Model file for the job. Use its own axes, mm. A direction names the side the tool comes from. Give positions to 0.01 mm unless a question says otherwise; leave off trailing zeros. Loops run counter-clockwise (first coordinate to the right, second up) from the corner with the lowest first, then second, coordinate; pieces in that order, holes last. Notation, with made-up numbers: (78, 11.5) - (85, 11.5) arc R26 ccw to (85, 31.5) - close; hole circle Ø11 at (11, 2). An arc over 180 degrees is marked (long way). Use a Markdown table: item, result.
from build123d import *

# Parameters (mm, degrees)
BOSS_EXTRUDE1_DEPTH         = 4.159999906
TAP_DRILL_FOR_M5X0_8_TAP1_D = 4.2
SKETCH8_W                   = 0.52
SKETCH8_H                   = 0.81


with BuildPart() as part:
    # Sketch1 → Boss-Extrude1 (new body)
    with BuildSketch(Plane(origin=(0, 0, 0), x_dir=(1, 0, 0), z_dir=(0, 1, 0))):
        Polygon((-4, -2.309401077), (0, -4.618802154), (4, -2.309401077), (4, 2.309401077), (0, 4.618802154), (-4, 2.309401077), align=None)
    extrude(amount=BOSS_EXTRUDE1_DEPTH)

    # Sketch3 → Revolve1 (revolve)
    with BuildSketch(Plane.XY):
        with BuildLine():
            Line((3.17, 4.989999906), (0, 4.989999906))
            Line((0, 4.989999906), (0, 4.159999906))
            Line((0, 4.159999906), (4, 4.159999906))
            ThreePointArc((4, 4.159999906), (3.756898628, 4.746898534), (3.17, 4.989999906))
        make_face()
    revolve(axis=Axis((0, 4.989999906, 0), (0, -1, 0)))

    # Tap Drill for M5x0.8 Tap1 (through all)
    with Locations(Plane(origin=(0, 0, 0), x_dir=(-1, 0, 0), z_dir=(0, -1, 0))):
        with Locations((0, 0)):
            Hole(TAP_DRILL_FOR_M5X0_8_TAP1_D / 2)

    # Sketch8 → Revolve2 (revolve)
    with BuildSketch(Plane.XY):
        with Locations((1.84, 4.554999966)):
            Rectangle(SKETCH8_W, SKETCH8_H)
    revolve(axis=Axis((0, 4.989999906, 0), (0, -1, 0)))


solid = part.part
(1) Pin check, flat tips, straight feed: P1, Ø0.6, axis at x = -3, z = -2, coming from the +Y side; P2, Ø2, axis at x = -2, y = 1, coming from the +Z side; P3, Ø1.3, axis at x = -0.5, z = 0.5, coming from the -Y side; P4, Ø0.9, axis at x = 0.5, z = 4, coming from the +Y side. Stop position of each tip, or through.
Computed:
| item | result |
|---|---|
| P1 | y = 4.98 |
| P2 | z = 4.04 |
| P3 | through |
| P4 | y = 4.88 |
(2) Slice it at A-A, the plane y = 1.5. Write the cut outline in (x, z), plus the area to 3 significant figures.
Computed:
| item | result |
|---|---|
| outline | (-4, -2.31) - (0, -4.62) - (4, -2.31) - (4, 2.31) - (0, 4.62) - (-4, 2.31) - close; hole circle Ø4.2 at (0, 0) |
| area | 41.6 mm² |
(3) Drill centre lines: probe 1 along X at (y, z) = (1.5, 0); probe 2 along Y at (x, z) = (-0.75, 1.5); probe 3 along Z at (x, y) = (-1.25, 2). Where is each one in solid material? Low to high. Write a range as [from, to].
Computed:
| item | result |
|---|---|
| probe 1 | [-4, -2.1], [2.1, 4] |
| probe 2 | [4.15, 4.96] |
| probe 3 | [-3.9, -1.69], [1.69, 3.9] |
(4) 3-axis set-ups, long thin cutter, end or side, ignore diameter. For faces 1 (the flat face through (-3.6, 4.16, 2.1)), 2 (the cylindrical face through (2.003, 2.104, -0.631)), 3 (the flat face through (3.6, 4.16, -2.1)), 4 (the flat face through (0, 4.16, 4.2)), 5 (the flat face through (-3.6, 4.16, -2.1)): which of +Z, -Z, +X, -X, +Y, -Y reach the whole face in a straight line?
Computed:
| item | result |
|---|---|
| face 1 | +Z, -X, +Y |
| face 2 | -Y |
| face 3 | -Z, +X, +Y |
| face 4 | +Z, +Y |
| face 5 | -Z, -X, +Y |
